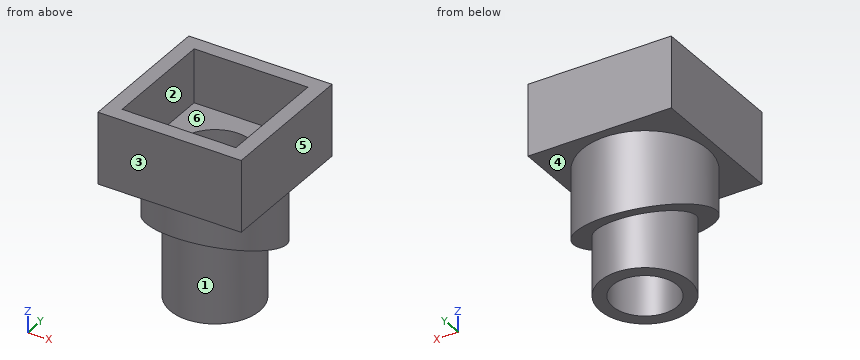
from build123d import *

# Parameters (mm, degrees)
CROQUIS1_R              = 2.5
CROQUIS1_R_2            = 1.8
SALIENTE_EXTRUIR1_DEPTH = 7
SALIENTE_EXTRUIR2_REACH = 9.842
CROQUIS3_R              = 3.5
CROQUIS3_R_2            = 1.6
CROQUIS4_W              = 8
CROQUIS4_H              = 8
CROQUIS4_R              = 2
SALIENTE_EXTRUIR3_DEPTH = 1
CROQUIS6_W              = 8
CROQUIS6_H              = 8
CROQUIS6_W_2            = 6.35
CROQUIS6_H_2            = 6.35
SALIENTE_EXTRUIR5_DEPTH = 3


with BuildPart() as part:
    # Croquis1 → Saliente-Extruir1 (new body)
    with BuildSketch(Plane.XY):
        Circle(CROQUIS1_R)
        Circle(CROQUIS1_R_2, mode=Mode.SUBTRACT)
    extrude(amount=SALIENTE_EXTRUIR1_DEPTH)

    # Saliente-Extruir2: up to this plane
    saliente_extruir2_end = Plane(origin=(0, 1.223696204, 3.362077689), z_dir=(0, -0.34202014332567576, -0.9396926207859059))
    # Croquis3 → Saliente-Extruir2 (add, up to the surface)
    with BuildSketch(Plane.XY.offset(7), mode=Mode.PRIVATE) as saliente_extruir2_sk1:
        Circle(CROQUIS3_R)
        Circle(CROQUIS3_R_2, mode=Mode.SUBTRACT)
    saliente_extruir2_tool1 = split(extrude(saliente_extruir2_sk1.sketch, amount=-SALIENTE_EXTRUIR2_REACH, mode=Mode.PRIVATE), bisect_by=saliente_extruir2_end, keep=Keep.BOTH, mode=Mode.PRIVATE)
    add(saliente_extruir2_tool1.solids().sort_by_distance((-3.401005, 0, 7))[0])

    # Croquis4 → Saliente-Extruir3 (add)
    with BuildSketch(Plane.XY.offset(7)):
        Rectangle(CROQUIS4_W, CROQUIS4_H)
        Circle(CROQUIS4_R, mode=Mode.SUBTRACT)
    extrude(amount=SALIENTE_EXTRUIR3_DEPTH)

    # Croquis6 → Saliente-Extruir5 (add)
    with BuildSketch(Plane.XY.offset(8)):
        Rectangle(CROQUIS6_W, CROQUIS6_H)
        Rectangle(CROQUIS6_W_2, CROQUIS6_H_2, mode=Mode.SUBTRACT)
    extrude(amount=SALIENTE_EXTRUIR5_DEPTH)


solid = part.part
The listing builds one solid part. Answer for the finished solid, in the listing's coordinates (mm). Face numbers are marked on the shaded views. A direction names the side the tool comes from. Round coordinates to 2 decimals unless told otherwise and drop trailing zeros. Order: outer loops, then holes, each group sorted by start corner. A loop starts at its lowest first (then second) coordinate and runs counter-clockwise, first axis right, second up. Notation, with made-up numbers: (36, -10) -> (69, -10) arc R17 cw to (69, 5) -> close; hole circle Ø10 at (40, 67.25). An arc over 180 degrees is marked (long way). Put each result on its own line as item: value.
Q1. Section D-D, the plane y = 2.25 is taken. Write down the section's boundary in (x, z) (3 decimals).
Results list:
outline: (-4, 7) -> (-2.681, 7) -> (-2.681, 2.989) -> (-1.09, 2.989) -> (-1.09, 0) -> (1.09, 0) -> (1.09, 2.989) -> (2.681, 2.989) -> (2.681, 7) -> (4, 7) -> (4, 11) -> (3.175, 11) -> (3.175, 8) -> (-3.175, 8) -> (-3.175, 11) -> (-4, 11) -> close
Q2. Section B-B, the plane x = 0.25 is taken. Write down the section's boundary in (y, z) (3 decimals), and give its area (3 significant figures).
Results list:
outline: (-4, 7) -> (-3.491, 7) -> (-3.491, 5.078) -> (-2.487, 4.713) -> (-2.487, 0) -> (-1.783, 0) -> (-1.783, 4.456) -> (-1.58, 4.383) -> (-1.58, 7) -> (-1.984, 7) -> (-1.984, 8) -> (-3.175, 8) -> (-3.175, 11) -> (-4, 11) -> close; (1.58, 3.232) -> (1.783, 3.159) -> (1.783, 0) -> (2.487, 0) -> (2.487, 2.902) -> (3.491, 2.537) -> (3.491, 7) -> (4, 7) -> (4, 11) -> (3.175, 11) -> (3.175, 8) -> (1.984, 8) -> (1.984, 7) -> (1.58, 7) -> close
area: 26.5 mm^2
Q3. Each of these flat-tipped pins is pushed along its axis until it touches: P1, Ø1, axis at x = -1, z = 1.5, coming from the -Y side; P2, Ø2.5, axis at x = 0, y = 0, coming from the +Z side; P3, Ø1, axis at x = 0.5, y = 3, coming from the -Z side; P4, Ø3.5, axis at x = 0, y = 0, coming from the -Z side. Where does it stop, or does it pass through?
Results list:
P1: y = -2.45
P2: through
P3: z = 2.54
P4: z = 3.17
Q4. Consider line 1 along X through (y, z) = (0, 1.8); line 2 along Y through (x, z) = (0, 7.45); line 3 along Y through (x, z) = (2.5, 8.5) (3 decimals). Determine where each line is inside the solid, lowest interval first.
Results list:
line 1: -2.5 to -1.8, 1.8 to 2.5
line 2: -4 to -2, 2 to 4
line 3: -4 to -3.175, 3.175 to 4
Q5. Section A-A, the plane y = 0 is taken. Write down the section's boundary in (x, z) (3 decimals), and give its area (3 significant figures).
Results list:
outline: (-4, 7) -> (-3.5, 7) -> (-3.5, 3.807) -> (-2.5, 3.807) -> (-2.5, 0) -> (-1.8, 0) -> (-1.8, 3.807) -> (-1.6, 3.807) -> (-1.6, 7) -> (-2, 7) -> (-2, 8) -> (-3.175, 8) -> (-3.175, 11) -> (-4, 11) -> close; (1.6, 3.807) -> (1.8, 3.807) -> (1.8, 0) -> (2.5, 0) -> (2.5, 3.807) -> (3.5, 3.807) -> (3.5, 7) -> (4, 7) -> (4, 11) -> (3.175, 11) -> (3.175, 8) -> (2, 8) -> (2, 7) -> (1.6, 7) -> close
area: 26.4 mm^2
Q6. Section C-C, the plane z = 9.5 is taken. Write down the section's boundary in (x, y) (3 decimals).
Results list:
outline: (-4, -4) -> (4, -4) -> (4, 4) -> (-4, 4) -> close; hole (-3.175, -3.175) -> (3.175, -3.175) -> (3.175, 3.175) -> (-3.175, 3.175) -> close
Q7. Which of the six approach directions +Z, -Z, +X, -X, +Y, -Y give full straight-line access (tool end or side, diameter ignored) to the marked faces 1, 2 and 3?
Results list:
face 1: -Z
face 2: +Z
face 3: +Z, -Z, +X, -X, -Y
Q8. Determine the mould class of the marked faces 4, 5 and 6 for opening direction Z: pulls with the +Z half, pulls with the -Z half, needs draft (parallel to the pull), parting line crosses it, or undercut.
Results list:
face 4: pulls with the -Z half
face 5: needs draft
face 6: pulls with the +Z half
